```python
from build123d import *

# Parameters (mm, degrees)
SKETCH1_R               = 1.65
BOSS_EXTRUDE1_DEPTH     = 3
SKETCH3_W               = 37
SKETCH3_H               = 24
BOSS_EXTRUDE3_DEPTH     = 6
CUT_EXTRUDE1_DEPTH      = 10
CUT_EXTRUDE1_DEPTH_BACK = 21
SKETCH4_R               = 1.65
CUT_EXTRUDE2_DEPTH      = 10
BOSS_EXTRUDE4_START     = -3
SKETCH7_R               = 1.65
BOSS_EXTRUDE4_DEPTH     = 3


with BuildPart() as part:
    # Sketch1 → Boss-Extrude1 (new body)
    with BuildSketch(Plane(origin=(0, 0, 0), x_dir=(1, 0, 0), z_dir=(0, 1, 0))):
        Polygon((-22.5, 0), (-18.5, 0), (-18.5, -42), (18.5, -42), (18.5, 0), (22.5, 0), (53, -37), (75, -37), (75, -24.590163934), (30, 30), (-30, 30), (-75, -24.590163934), (-75, -37), (-53, -37), align=None)
        with Locations(Location((70.5, -32, 0), (0, 0, 270))):
            Circle(SKETCH1_R, mode=Mode.SUBTRACT)
        with Locations(Location((-70.5, -32, 0), (0, 0, 270))):
            Circle(SKETCH1_R, mode=Mode.SUBTRACT)
    extrude(amount=BOSS_EXTRUDE1_DEPTH)

    # Sketch3 → Boss-Extrude3 (add)
    with BuildSketch(Plane(origin=(0, 0, 0), x_dir=(1, 0, 0), z_dir=(0, 1, 0))):
        with Locations((0, -30)):
            Rectangle(SKETCH3_W, SKETCH3_H)
    extrude(amount=-BOSS_EXTRUDE3_DEPTH)

    # Sketch4 → Cut-Extrude1 (cut, two sides: drawn at the far end of the back side and taken through both)
    with BuildSketch(Plane(origin=(0, 0, 0), x_dir=(1, 0, 0), z_dir=(0, 1, 0)).offset(-CUT_EXTRUDE1_DEPTH_BACK)):
        with Locations(Location((-11, -35, 0), (0, 0, 270))):
            Circle(SKETCH4_R)
        with Locations(Location((11, -35, 0), (0, 0, 270))):
            Circle(SKETCH4_R)
        with Locations(Location((-11, -25, 0), (0, 0, 270))):
            Circle(SKETCH4_R)
        with Locations(Location((11, -25, 0), (0, 0, 270))):
            Circle(SKETCH4_R)
    extrude(amount=CUT_EXTRUDE1_DEPTH + CUT_EXTRUDE1_DEPTH_BACK, mode=Mode.SUBTRACT)

    # Sketch5 → Cut-Extrude2 (cut)
    with BuildSketch(Plane(origin=(0, 0, 0), x_dir=(1, 0, 0), z_dir=(0, 1, 0))):
        with BuildLine():
            ThreePointArc((-15, 0), (-12, 3), (-15, 6))
            ThreePointArc((-15, 6), (-18, 3), (-15, 0))
        make_face()
    extrude(amount=CUT_EXTRUDE2_DEPTH, mode=Mode.SUBTRACT)

    # Sketch7 → Boss-Extrude4 (add)
    # profile 1 of 2: a face of its own
    with BuildSketch(Plane(origin=(0, 0, 0), x_dir=(1, 0, 0), z_dir=(0, 1, 0)).offset(BOSS_EXTRUDE4_START)):
        Polygon((65, -12.459016393), (65, -37), (75, -37), (75, -24.590163934), align=None)
        with Locations(Location((70.5, -32, 0), (0, 0, 270))):
            Circle(SKETCH7_R, mode=Mode.SUBTRACT)
    # profile 2 of 2: a face of its own
    with BuildSketch(Plane(origin=(0, 0, 0), x_dir=(1, 0, 0), z_dir=(0, 1, 0)).offset(BOSS_EXTRUDE4_START)):
        Polygon((-75, -24.590163934), (-65, -12.459016393), (-65, -37), (-75, -37), align=None)
        with Locations(Location((-70.5, -32, 0), (0, 0, 270))):
            Circle(SKETCH7_R, mode=Mode.SUBTRACT)
    extrude(amount=BOSS_EXTRUDE4_DEPTH)


solid = part.part
```
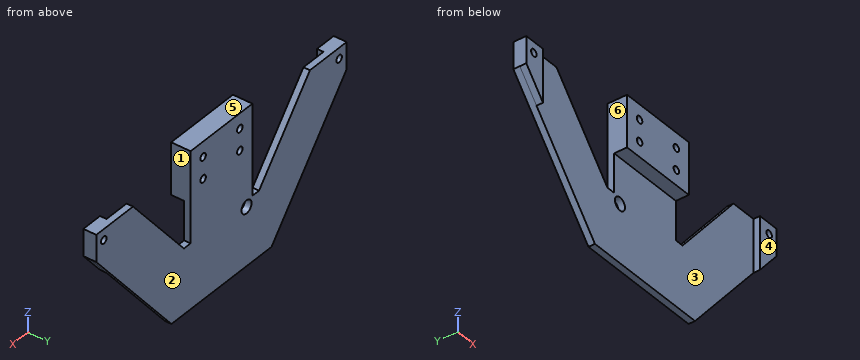
Part model, mm, in its own coordinate system. Face numbers are marked on the shaded views. A direction names the side the tool comes from. Give positions to 0.01 mm unless a question says otherwise; leave off trailing zeros. Write each loop counter-clockwise with the first axis right and the second up, starting at its lowest first coordinate (ties: lowest second). Pieces come first, ordered by that corner, then holes. Notation, with made-up numbers: (-13, 87.5) -> (28, 87.5) arc R8 ccw to (28, 91.5) -> close; hole circle Ø10 at (73, 57.25). An arc over 180 degrees is marked (long way). Put each result on its own line as item: value. Start each with the question number.
Item 1: Wall check: L1, parallel to Z at x = -11, y = 0.75; L2, parallel to Z at x = -11, y = -2.25; L3, parallel to X at y = -0.25, z = 35. Give the ranges that are in metal, low to high. Write a range as [from, to].
Item 2: Pull direction X, two halves, no side cores. Call the marked faces 5 and 6: pulls with the +X half, pulls with the -X half, needs draft (parallel to the pull), parting line crosses it, or undercut.
Item 3: Which spindle directions (+Z, -Z, +X, -X, +Y, -Y) get a long thin tool onto all of the face, cutting with end or side? Do the marked faces 1, 2, 3 and 4. Say none if no direction does.
Item 4: Cut at D-D (z = 35). List the corners of the cut face in (x, y).
Item 5: Cut at B-B (x = 11). List the corners of the cut face in (y, z).
Item 6: Cut at C-C (x = -15). List the corners of the cut face in (y, z).
Item 7: Pin check, flat tips, straight feed: pin 1 Ø7 at (x, z) = (-15, -3) entering from -Y; pin 2 Ø3 at (y, z) = (0.5, -2.5) entering from -X; pin 3 Ø2 at (x, z) = (11, 35) entering from -Y; pin 4 Ø5 at (x, y) = (-49.5, -1.5) entering from +Z. Stop position of each tip, or through.
Item 8: Cut at A-A (y = -1.5). State how many separate pieces and enclosed holes the cut face has, then the cut area to 3 significant figures.
Answer list:
1. L1: z = [-30, 23.35], [26.65, 33.35], [36.65, 42]
1. L2: z = [18, 23.35], [26.65, 33.35], [36.65, 42]
1. L3: x = [-75, -65], [-18.5, -12.65], [-9.35, 9.35], [12.65, 18.5], [65, 75]
2. face 5: needs draft
2. face 6: undercut
3. face 1: +Z, +Y, -Y
3. face 2: +Z, -Z, +X, -X, +Y
3. face 3: -Z, -Y
3. face 4: +Z, -Z, +X, -Y
4. outline: (-75, -3) -> (-65, -3) -> (-65, 0) -> (-51.35, 0) -> (-51.35, 3) -> (-75, 3) -> close; (-18.5, -6) -> (-12.65, -6) -> (-12.65, 3) -> (-18.5, 3) -> close; (-9.35, -6) -> (9.35, -6) -> (9.35, 3) -> (-9.35, 3) -> close; (12.65, -6) -> (18.5, -6) -> (18.5, 3) -> (12.65, 3) -> close; (51.35, 0) -> (65, 0) -> (65, -3) -> (75, -3) -> (75, 3) -> (51.35, 3) -> close
5. outline: (-6, 18) -> (0, 18) -> (0, -30) -> (3, -30) -> (3, 23.35) -> (-6, 23.35) -> close; (-6, 26.65) -> (3, 26.65) -> (3, 33.35) -> (-6, 33.35) -> close; (-6, 36.65) -> (3, 36.65) -> (3, 42) -> (-6, 42) -> close
6. outline: (-6, 18) -> (0, 18) -> (0, 0) -> (3, 0) -> (3, 42) -> (-6, 42) -> close; (0, -30) -> (3, -30) -> (3, -6) -> (0, -6) -> close
7. pin 1: stops at y = 0
7. pin 2: stops at x = -53.91
7. pin 3: passes through
7. pin 4: stops at z = 35.18
8. separate pieces: 3
8. enclosed holes: 6
8. area: 1,210 mm2
